Check sheet for the modelled part. Datum: model origin and axes. Units: mm. A direction names the side the tool comes from. Give positions to 0.01 mm unless a question says otherwise; leave off trailing zeros. Write each loop counter-clockwise with the first axis right and the second up, starting at its lowest first coordinate (ties: lowest second). Pieces come first, ordered by that corner, then holes. Notation, with made-up numbers: M 57.5,0 L 79.5,0 A21 cw 79.5,24 Z; hole C 48,0 d7. An arc over 180 degrees is marked long. Write each question's results on one line, items separated by ' | '. Start each with the question number.
from build123d import *

# Parameters (mm, degrees)
BOSS_EXTRU_1_DEPTH      = 6.35
ESQUISSE2_W             = 18.18
ESQUISSE2_H             = 6.35
ESQUISSE2_W_2           = 6.35
ESQUISSE2_H_2           = 18.181818182
ESQUISSE2_W_3           = 18.181818182
ENL_V_MAT_EXTRU_1_DEPTH = 6.35


with BuildPart() as part:
    # Esquisse1 → Boss.-Extru.1 (new body)
    with BuildSketch(Plane(origin=(0, 0, 0), x_dir=(1, 0, 0), z_dir=(0, 1, 0))):
        with BuildLine():
            Line((0, -82.5), (0, -100))
            Line((0, -100), (-100, -100))
            Line((-100, -100), (-100, 100))
            Line((-100, 100), (0, 100))
            Line((0, 100), (0, 82.5))
            ThreePointArc((0, 82.5), (-82.5, 0), (0, -82.5))
        make_face()
    extrude(amount=BOSS_EXTRU_1_DEPTH)

    # Esquisse2 → Enlèv. mat.-Extru.1 (cut)
    with BuildSketch(Plane(origin=(0, 6.35, 0), x_dir=(1, 0, 0), z_dir=(0, 1, 0))):
        with Locations((-72.73, -96.825)):
            Rectangle(ESQUISSE2_W, ESQUISSE2_H)
        with Locations((-36.37, -96.825)):
            Rectangle(ESQUISSE2_W, ESQUISSE2_H)
        with Locations((-0.01, -96.825)):
            Rectangle(ESQUISSE2_W, ESQUISSE2_H)
        with Locations((-96.825, -72.727272727)):
            Rectangle(ESQUISSE2_W_2, ESQUISSE2_H_2)
        with Locations((-96.825, -36.363636364)):
            Rectangle(ESQUISSE2_W_2, ESQUISSE2_H_2)
        with Locations((-96.825, 0)):
            Rectangle(ESQUISSE2_W_2, ESQUISSE2_H_2)
        with Locations((-96.825, 36.363636364)):
            Rectangle(ESQUISSE2_W_2, ESQUISSE2_H_2)
        with Locations((-96.825, 72.727272727)):
            Rectangle(ESQUISSE2_W_2, ESQUISSE2_H_2)
        with Locations((-72.727272727, 96.825)):
            Rectangle(ESQUISSE2_W_3, ESQUISSE2_H)
        with Locations((-36.363636364, 96.825)):
            Rectangle(ESQUISSE2_W_3, ESQUISSE2_H)
        with Locations((-0.000909091, 96.825)):
            Rectangle(ESQUISSE2_W, ESQUISSE2_H)
    extrude(amount=-ENL_V_MAT_EXTRU_1_DEPTH, mode=Mode.SUBTRACT)


solid = part.part
Q1. Tool access check on faces 1 (the face through (-73, 3, -93.65)), 2 (the face through (-97, 3, -45.455)), 3 (the face through (-9.1, 3, 97)), 4 (the face through (-81.82, 3, 97)), 5 (the face through (-9.091, 3, -97)). Record the directions out of +Z, -Z, +X, -X, +Y, -Y that give a thin tool (end or side, any length) a straight path to the whole face; none if there is none.
Q2. Section check A-A on x = -71.5. Record the boundary of the cut face in (y, z).
Q3. Release check for a two-part mould opening along X. For faces 6 (the face through (-63.64, 3, 97)), 7 (the face through (-100, 3, -91)), 8 (the face through (-91, 3, 100)), 9 (the face through (-45.46, 3, 97)) record: pulls with the +X half, pulls with the -X half, needs draft (parallel to the pull), parting line crosses it, or undercut.
Q4. Scan lines: L1, parallel to Z at x = -94, y = 4.75; L2, parallel to Z at x = -19.5, y = 3.75; L3, parallel to Z at x = -16.5, y = 3.25. Record each from-to range of solid material in increasing order.
Q5. Section check C-C on z = -49.5. Record the boundary of the cut face in (x, y).
Q6. Section check B-B on z = 0. Record the boundary of the cut face in (x, y).
Q7. Depth check by flat-ended pin: pin 1 Ø3 at (y, z) = (3.5, -37) entering from -X; pin 2 Ø3 at (y, z) = (4.5, 98) entering from +X; pin 3 Ø1.9 at (x, y) = (-33, 4) entering from -Z. Enter the tip coordinate at first touch or a pass-through.
Check result:
1) face 1: -Z, +Y, -Y | face 2: -X, +Y, -Y | face 3: +Z, +X, +Y, -Y | face 4: +Z, +Y, -Y | face 5: -Z, +X, +Y, -Y
2) outline: M 0,-93.65 L 6.35,-93.65 L 6.35,-41.16 L 0,-41.16 Z; M 0,41.16 L 6.35,41.16 L 6.35,93.65 L 0,93.65 Z
3) face 6: undercut | face 7: pulls with the -X half | face 8: needs draft | face 9: undercut
4) L1: -100 to -81.82, -63.64 to -45.45, -27.27 to -9.09, 9.09 to 27.27, 45.45 to 63.64, 81.82 to 100 | L2: -100 to -80.16, 80.16 to 100 | L3: -100 to -80.83, 80.83 to 100
5) outline: M -100,0 L -66,0 L -66,6.35 L -100,6.35 Z
6) outline: M -93.65,0 L -82.5,0 L -82.5,6.35 L -93.65,6.35 Z
7) pin 1: x = -93.65 | pin 2: x = -9.1 | pin 3: z = -93.65
